```python
from build123d import *

# Parameters (mm, degrees)
F0_W     = 101.6
F0_H     = 50.8
F1_DEPTH = 25.4
F2_W     = 50.8
F2_H     = 38.1
F3_DEPTH = 25.4
F5_DEPTH = 38.1
F6_R     = 6.35
F7_DEPTH = 50.8
F8_R     = 6.35
F9_DEPTH = 25.4


with BuildPart() as f1:
    # F0 (on Front) → F1 (new body)
    with BuildSketch(Plane.XZ):
        with Locations((-24.0954693718, 25.4)):
            Rectangle(F0_W, F0_H)
    extrude(amount=F1_DEPTH)

    # F2 (on face) → F3 (cut)
    with BuildSketch(Plane.XZ.offset(25.4)):
        with Locations((1.3045306282, 31.75)):
            Rectangle(F2_W, F2_H)
    extrude(amount=-F3_DEPTH, mode=Mode.SUBTRACT)

    # F4 (on face) → F5 (cut)
    with BuildSketch(Plane.XY.offset(50.8)):
        Polygon((-49.4954693718, -25.4), (-49.4954693718, -12.7), (-49.4954693718, 0), (-74.8954693718, 0), (-74.8954693718, -25.4), align=None)
        with BuildLine():
            Line((-24.0954693718, -25.4), (-24.0954693718, -12.7))
            ThreePointArc((-24.0954693718, -12.7), (-27.8152132507, -21.6802561211), (-36.7954693718, -25.4))
            Line((-36.7954693718, -25.4), (-24.0954693718, -25.4))
        make_face()
        with BuildLine():
            ThreePointArc((-36.7954693718, 0), (-27.8152132507, -3.7197438789), (-24.0954693718, -12.7))
            Line((-24.0954693718, -12.7), (-24.0954693718, 0))
            Line((-24.0954693718, 0), (-36.7954693718, 0))
        make_face()
        with BuildLine():
            Line((-49.4954693718, -25.4), (-36.7954693718, -25.4))
            ThreePointArc((-36.7954693718, -25.4), (-45.7757254928, -21.6802561211), (-49.4954693718, -12.7))
            Line((-49.4954693718, -12.7), (-49.4954693718, -25.4))
        make_face()
        with BuildLine():
            ThreePointArc((-49.4954693718, -12.7), (-45.7757254928, -3.7197438789), (-36.7954693718, 0))
            Line((-36.7954693718, 0), (-49.4954693718, 0))
            Line((-49.4954693718, 0), (-49.4954693718, -12.7))
        make_face()
    extrude(amount=-F5_DEPTH, mode=Mode.SUBTRACT)

    # F6 (on face) → F7 (cut)
    with BuildSketch(Plane.XY.offset(50.8)):
        with Locations((-36.7954693718, -12.7)):
            Circle(F6_R)
    extrude(amount=-F7_DEPTH, mode=Mode.SUBTRACT)

    # F8 (on Top) → F9 (cut)
    with BuildSketch(Plane.XY):
        with Locations((-62.1954693718, -12.7)):
            Circle(F8_R)
        with BuildLine():
            ThreePointArc((-11.3954693718, -19.05), (-6.9053413112, -17.1901280605), (-5.0454693718, -12.7))
            ThreePointArc((-5.0454693718, -12.7), (-6.9053413112, -8.2098719395), (-11.3954693718, -6.35))
            ThreePointArc((-11.3954693718, -6.35), (-17.7454693718, -12.7), (-11.3954693718, -19.05))
        make_face()
        with BuildLine():
            ThreePointArc((-11.3954693718, -6.35), (-6.9053413112, -8.2098719395), (-5.0454693718, -12.7))
            ThreePointArc((-5.0454693718, -12.7), (-6.9053413112, -17.1901280605), (-11.3954693718, -19.05))
            Line((-11.3954693718, -19.05), (14.0045306282, -19.05))
            ThreePointArc((14.0045306282, -19.05), (7.6545306282, -12.7), (14.0045306282, -6.35))
            Line((14.0045306282, -6.35), (-11.3954693718, -6.35))
        make_face()
        with BuildLine():
            ThreePointArc((20.3545306282, -12.7), (18.4946586888, -8.2098719395), (14.0045306282, -6.35))
            ThreePointArc((14.0045306282, -6.35), (7.6545306282, -12.7), (14.0045306282, -19.05))
            ThreePointArc((14.0045306282, -19.05), (18.4946586888, -17.1901280605), (20.3545306282, -12.7))
        make_face()
        with BuildLine():
            Line((-74.8954693718, 0), (-74.8954693718, -12.7))
            ThreePointArc((-74.8954693718, -12.7), (-71.1757254928, -3.7197438789), (-62.1954693718, 0))
            Line((-62.1954693718, 0), (-74.8954693718, 0))
        make_face()
        with BuildLine():
            ThreePointArc((-62.1954693718, -25.4), (-71.1757254928, -21.6802561211), (-74.8954693718, -12.7))
            Line((-74.8954693718, -12.7), (-74.8954693718, -25.4))
            Line((-74.8954693718, -25.4), (-62.1954693718, -25.4))
        make_face()
        with BuildLine():
            Line((26.7045306282, -25.4), (26.7045306282, -12.7))
            ThreePointArc((26.7045306282, -12.7), (22.9847867493, -21.6802561211), (14.0045306282, -25.4))
            Line((14.0045306282, -25.4), (26.7045306282, -25.4))
        make_face()
        with BuildLine():
            ThreePointArc((14.0045306282, 0), (22.9847867493, -3.7197438789), (26.7045306282, -12.7))
            Line((26.7045306282, -12.7), (26.7045306282, 0))
            Line((26.7045306282, 0), (14.0045306282, 0))
        make_face()
    extrude(amount=F9_DEPTH, mode=Mode.SUBTRACT)


solid = f1.part
```
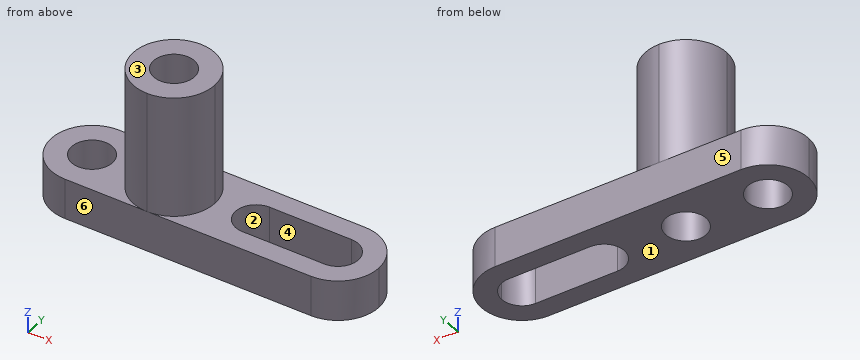
Source: CAD feature listing. Evaluate the final solid. Frame: model axes, mm. Face numbers are marked on the shaded views. A direction names the side the tool comes from. Round coordinates to 2 decimals unless told otherwise and drop trailing zeros. Order: outer loops, then holes, each group sorted by start corner. A loop starts at its lowest first (then second) coordinate and runs counter-clockwise, first axis right, second up. Notation, with made-up numbers: (86, 61) -> (97, 61) arc R20 ccw to (97, 86) -> close; hole circle Ø11 at (28.5, 12.5). An arc over 180 degrees is marked (long way). One line per item, written item: value. Start each with the question number.
Q1. Draft query along Y for the marked faces 3, 4, 5 and 6. Return one class per face: pulls with the +Y half, pulls with the -Y half, needs draft (parallel to the pull), parting line crosses it, or undercut.
Q2. Material intervals for probe 1 along X at (y, z) = (-12.75, 34.5); probe 2 along Z at (x, y) = (-21, -16.75); probe 3 along Y at (x, z) = (3.5, 6.5), sorted ascending.
Q3. Section query C-C (x = -67). Return the cut outline in (y, z), plus the area to 3 significant figures.
Q4. Section query A-A (y = -11.75). Return the cut outline in (x, z), plus the area to 3 significant figures.
Q5. Access query for the marked faces 1 and 2. Directions: +Z, -Z, +X, -X, +Y, -Y. A direction counts if a zero-diameter tool reaches every point of the face in a straight line with its end or side. Return the directions, or none.
Q6. Section query D-D (y = -4.5). Return the cut outline in (x, z).
Q7. Pin query (flat end, axial travel): pin 1 (3 mm diameter, centred on y = -22.5, z = 16.5, fed in from +X); pin 2 (8 mm diameter, centred on y = -13.5, z = 27, fed in from +X); pin 3 (11.5 mm diameter, centred on x = -62.2, y = -12.7, fed in from +Z). Return the tip coordinate at first contact, or that it passes through.
Q8. Section query B-B (z = 19.5). Return the cut outline in (x, y), plus the area to 3 significant figures.
Findings below:
1. face 3: needs draft
1. face 4: undercut
1. face 5: pulls with the +Y half
1. face 6: pulls with the -Y half
2. probe 1: -49.5 to -43.15, -30.45 to -24.1
2. probe 2: 0 to 12.7
2. probe 3: -25.4 to -19.05, -6.35 to 0
3. outline: (-24.46, 0) -> (-16.85, 0) -> (-16.85, 12.7) -> (-24.46, 12.7) -> close; (-8.55, 0) -> (-0.94, 0) -> (-0.94, 12.7) -> (-8.55, 12.7) -> close
3. area: 193 mm²
4. outline: (-74.86, 0) -> (-68.47, 0) -> (-68.47, 12.7) -> (-74.86, 12.7) -> close; (-55.92, 0) -> (-43.07, 0) -> (-43.07, 50.8) -> (-49.46, 50.8) -> (-49.46, 12.7) -> (-55.92, 12.7) -> close; (-30.52, 0) -> (-17.67, 0) -> (-17.67, 12.7) -> (-24.13, 12.7) -> (-24.13, 50.8) -> (-30.52, 50.8) -> close; (20.28, 0) -> (26.67, 0) -> (26.67, 12.7) -> (20.28, 12.7) -> close
4. area: 975 mm²
5. face 1: -Z, +X, -X, +Y, -Y
5. face 2: +Z, -Z
6. outline: (-71.89, 0) -> (23.7, 0) -> (23.7, 12.7) -> (-27.1, 12.7) -> (-27.1, 50.8) -> (-46.49, 50.8) -> (-46.49, 12.7) -> (-71.89, 12.7) -> close
7. pin 1: x = -27.18
7. pin 2: x = -24.1
7. pin 3: through
8. outline: circle Ø25.4 at (-36.8, -12.7); hole circle Ø12.7 at (-36.8, -12.7)
8. area: 380 mm²
